from build123d import *

# Parameters (mm, degrees)
EXTRUDE_5_DEPTH      = 30
EXTRUDE_5_DEPTH_BACK = 30
F_1_FR_R             = 5
EXTRUDE_6_DEPTH      = 20
EXTRUDE_6_DEPTH_BACK = 20


with BuildPart() as part:
    # Эскиз1_fr → Бобышка-Вытянуть5 (new, two sides: drawn at the far end of the back side and taken through both)
    with BuildSketch(Plane.XY.offset(-EXTRUDE_5_DEPTH_BACK)):
        with BuildLine():
            Line((-5.557606452, -13.932444528), (-5.557606452, -62.642280008))
            Line((-5.557606452, -62.642280008), (5.557606452, -62.642280008))
            Line((5.557606452, -62.642280008), (5.557606452, -13.932444528))
            ThreePointArc((5.557606452, -13.932444528), (0, 15), (-5.557606452, -13.932444528))
        make_face()
        Circle(F_1_FR_R, mode=Mode.SUBTRACT)
    extrude(amount=EXTRUDE_5_DEPTH + EXTRUDE_5_DEPTH_BACK)


with BuildPart() as body_2:
    # Эскиз3 → Бобышка-Вытянуть6 (new, two sides: drawn at the far end of the back side and taken through both)
    with BuildSketch(Plane(origin=(0, 0, 0), x_dir=(0, 0, -1), z_dir=(1, 0, 0)).offset(-EXTRUDE_6_DEPTH_BACK)):
        Polygon((-58.394498043, -50.25314581), (-85.938130262, -50.25314581), (-85.938130262, 27.580465306), (-80.938130262, 27.580465306), (-80.938130262, -45.25314581), (-63.394498043, -45.25314581), (-63.394498043, 27.580465306), (-58.394498043, 27.580465306), align=None)
    extrude(amount=EXTRUDE_6_DEPTH + EXTRUDE_6_DEPTH_BACK)


with BuildPart() as body_2_1:
    # Move Body 1: moved
    add(body_2.part.moved(Location((0, 0, -70))))


with BuildPart() as part_1:
    add(part.part)

    # Combine 1: intersect body 2
    add(body_2_1.part, mode=Mode.INTERSECT)


solid = part_1.part
Read the model definition and answer for the solid it produces. Units are mm, in the model's axes. A direction names the side the tool comes from. Give positions to 0.01 mm unless a question says otherwise; leave off trailing zeros. Write each loop counter-clockwise with the first axis right and the second up, starting at its lowest first coordinate (ties: lowest second). Pieces come first, ordered by that corner, then holes. Notation, with made-up numbers: (-36.5, 42) - (0.5, 42) arc R21 ccw to (0.5, 62) - close; hole circle Ø10 at (-27, 64.25). An arc over 180 degrees is marked (long way). Answer in a Markdown table with one row per item. Add a question column.
Item 1: A tool of negligible diameter and unlimited length cuts with its end or side. For faces 4 (the face through (-5.558, -32, -7)), 5 (the face through (0, -8, 10.938)), 6 (the face through (-1.08, -4.88, 13.4)), 7 (the face through (5.558, -32, -7)), 8 (the face through (0, -50.253, 2)), from which of +Z, -Z, +X, -X, +Y, -Y can it reach the whole face along a straight path? Write none if from no direction.
Item 2: Section C-C, the plane y = -25 is taken. Write down the section's boundary in (x, z), and give its area (3 significant figures).
Item 3: Determine the mould class of faces 1 (the face through (0, -10, -11.606)), 2 (the face through (0, -9, -6.606)), 3 (the face through (0.58, 14.99, -9.14)) for opening direction Z: pulls with the +Z half, pulls with the -Z half, needs draft (parallel to the pull), parting line crosses it, or undercut.
Item 4: Flat-ended cylindrical pins translate along their axes: P1, Ø11.5, axis at x = 0, y = 0, coming from the +Z side; P2, Ø6, axis at y = -34, z = -7, coming from the -X side; P3, Ø1, axis at y = -14, z = 12.5, coming from the +X side; P4, Ø1, axis at x = -9, z = -7.5, coming from the -Y side. Find the tip coordinate at first contact, or state that the pin passes through.
Item 5: Section D-D, the plane z = 9 is taken. Write down the section's boundary in (x, y), and give its area (3 significant figures).
Item 6: Find the intervals of material crossed by L1, parallel to Z at x = -9.5, y = 6; L2, parallel to Y at x = 0, z = 14.8; L3, parallel to X at y = 0, z = 14.05, in increasing order.
Item 7: Section A-A, the plane x = 0 is taken. Write down the section's boundary in (y, z), and give its area (3 significant figures).
Item 8: Section B-B, the plane y = 0 is taken. Write down the section's boundary in (x, z).
Recorded:
| question | item | result |
|---|---|---|
| 1 | face 4 | +Z, -Z, -X, -Y |
| 1 | face 5 | +X, -X, +Y |
| 1 | face 6 | +Z, -Z |
| 1 | face 7 | +Z, -Z, +X, -Y |
| 1 | face 8 | +Z, -Z, +X, -X, -Y |
| 2 | outline | (-5.56, -11.61) - (5.56, -11.61) - (5.56, -6.61) - (-5.56, -6.61) - close; (-5.56, 10.94) - (5.56, 10.94) - (5.56, 15.94) - (-5.56, 15.94) - close |
| 2 | area | 111 mm2 |
| 3 | face 1 | pulls with the -Z half |
| 3 | face 2 | undercut |
| 3 | face 3 | needs draft |
| 4 | P1 | stops at z = 15.94 |
| 4 | P2 | stops at x = -5.56 |
| 4 | P3 | stops at x = 6.54 |
| 4 | P4 | stops at y = -12.36 |
| 5 | outline | (-5.56, -50.25) - (5.56, -50.25) - (5.56, -45.25) - (-5.56, -45.25) - close |
| 5 | area | 55.6 mm2 |
| 6 | L1 | z = -11.61 to -6.61, 10.94 to 15.94 |
| 6 | L2 | y = -50.25 to -5, 5 to 15 |
| 6 | L3 | x = -15 to -5, 5 to 15 |
| 7 | outline | (-50.25, -11.61) - (-5, -11.61) - (-5, -6.61) - (-45.25, -6.61) - (-45.25, 10.94) - (-5, 10.94) - (-5, 15.94) - (-50.25, 15.94) - close; (5, -11.61) - (15, -11.61) - (15, -6.61) - (5, -6.61) - close; (5, 10.94) - (15, 10.94) - (15, 15.94) - (5, 15.94) - close |
| 7 | area | 640 mm2 |
| 8 | outline | (-15, -11.61) - (-5, -11.61) - (-5, -6.61) - (-15, -6.61) - close; (-15, 10.94) - (-5, 10.94) - (-5, 15.94) - (-15, 15.94) - close; (5, -11.61) - (15, -11.61) - (15, -6.61) - (5, -6.61) - close; (5, 10.94) - (15, 10.94) - (15, 15.94) - (5, 15.94) - close |
